Model file for the job. Use its own axes, mm. Give positions to 0.01 mm unless a question says otherwise; leave off trailing zeros. Loops run counter-clockwise (first coordinate to the right, second up) from the corner with the lowest first, then second, coordinate; pieces in that order, holes last. Notation, with made-up numbers: M -18,38.5 L 24,38.5 A13 cw 24,58.5 Z; hole C -8,16.25 d7. An arc over 180 degrees is marked long. Answer in a Markdown table with one row per item.
```python
from build123d import *

# Parameters (mm, degrees)
SKETCH_1_W          = 20
SKETCH_1_H          = 20
SKETCH_1_W_2        = 17
SKETCH_1_H_2        = 17
EXTRUDE_1_DEPTH     = 325.04
SKETCH_4_R          = 1.6
CUT_EXTRUDE_3_DEPTH = 326.808228257
SKETCH_6_R          = 1.5
CUT_EXTRUDE_5_DEPTH = 326.808228257


with BuildPart() as part:
    # 草图1 → 凸台-拉伸1 (new body)
    with BuildSketch(Plane.XY):
        Rectangle(SKETCH_1_W, SKETCH_1_H)
        Rectangle(SKETCH_1_W_2, SKETCH_1_H_2, mode=Mode.SUBTRACT)
    extrude(amount=EXTRUDE_1_DEPTH)

    # 草图4 → 切除-拉伸3 (cut, through all)
    with BuildSketch(Plane.ZY.offset(10)):
        with Locations(Location((282.54, 0, 0), (0, 0, 270))):
            Circle(SKETCH_4_R)
        with Locations(Location((302.54, 0, 0), (0, 0, 270))):
            Circle(SKETCH_4_R)
    extrude(amount=-CUT_EXTRUDE_3_DEPTH, mode=Mode.SUBTRACT)

    # 草图6 → 切除-拉伸5 (cut, through all)
    with BuildSketch(Plane(origin=(0, 10, 0), x_dir=(1, 0, 0), z_dir=(0, 1, 0))):
        with Locations(Location((0, -10, 0), (0, 0, 270))):
            Circle(SKETCH_6_R)
        with Locations(Location((0, -30, 0), (0, 0, 270))):
            Circle(SKETCH_6_R)
        with Locations(Location((0, -50, 0), (0, 0, 270))):
            Circle(SKETCH_6_R)
        with Locations(Location((0, -70, 0), (0, 0, 270))):
            Circle(SKETCH_6_R)
        with Locations(Location((0, -90, 0), (0, 0, 270))):
            Circle(SKETCH_6_R)
        with Locations(Location((0, -110, 0), (0, 0, 270))):
            Circle(SKETCH_6_R)
        with Locations(Location((0, -130, 0), (0, 0, 270))):
            Circle(SKETCH_6_R)
        with Locations(Location((0, -150, 0), (0, 0, 270))):
            Circle(SKETCH_6_R)
    extrude(amount=-CUT_EXTRUDE_5_DEPTH, mode=Mode.SUBTRACT)


solid = part.part
```
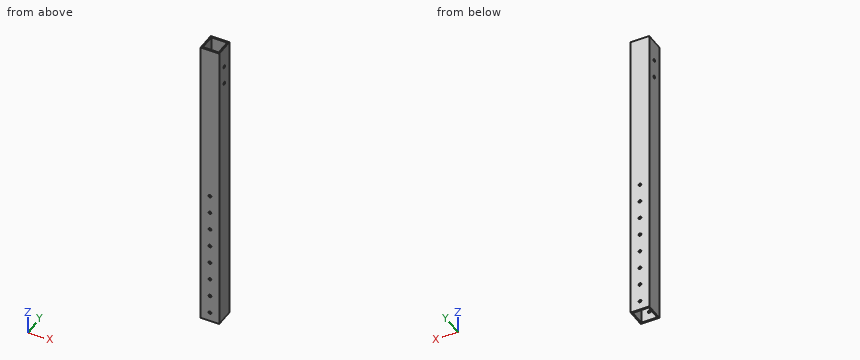
(1) Saw through at A-A, the plane x = -5.5. Give the cut face in (y, z).
Established:
| item | result |
|---|---|
| outline | M -10,0 L -8.5,0 L -8.5,325.04 L -10,325.04 Z; M 8.5,0 L 10,0 L 10,325.04 L 8.5,325.04 Z |
(2) Saw through at C-C, the plane z = 156. Give the cut face in (x, y), and give its area (3 significant figures).
Established:
| item | result |
|---|---|
| outline | M -10,-10 L 10,-10 L 10,10 L -10,10 Z; hole M -8.5,-8.5 L 8.5,-8.5 L 8.5,8.5 L -8.5,8.5 Z |
| area | 111 mm2 |
(3) Wall check: L1, parallel to X at y = -8, z = 147; L2, parallel to X at y = -8.95, z = 130. Give the ranges that are in metal, low to high.
Established:
| item | result |
|---|---|
| L1 | x = -10 to -8.5, 8.5 to 10 |
| L2 | x = -10 to -1.5, 1.5 to 10 |
(4) Flat gauge pin, fed straight in: P1, Ø1.8, axis at x = 0, z = 130, coming from the -Y side. Where does the tip first touch, or does it go through?
Established:
| item | result |
|---|---|
| P1 | passes through |
